Job drawing, mm, ordinate dimensions from the low corner. One solid piece. A direction names the side the tool comes from. Round coordinates to 2 decimals unless told otherwise and drop trailing zeros. Write each loop counter-clockwise with the first axis right and the second up, starting at its lowest first coordinate (ties: lowest second). Pieces come first, ordered by that corner, then holes.
1) Which spindle directions (+Z, -Z, +X, -X, +Y, -Y) get a long thin tool onto all of the face, cutting with end or side? Do the marked faces 1 and 2. Say none if no direction does.
2) Saw through at A-A on z = 20.2. Write the cut outline in (x, y), and give its area (3 significant figures).
3) Saw through at D-D on x = 1.75. Write the cut outline in (y, z), and give its area (3 significant figures).
4) Saw through at B-B on x = 10.75. Write the cut outline in (y, z), and give its area (3 significant figures).
5) Saw through at C-C on z = 9.25. Write the cut outline in (x, y), and give its area (3 significant figures).
6) Drill centre lines: L1, parallel to Z at x = 11, y = 0.9; L2, parallel to X at y = 0.2, z = 5.2; L3, parallel to Y at x = 13.5, z = 4.75. Where is each one in solid material? Low to high.
7) Flat gauge pins, fed straight in: pin 1 (1.1 mm diameter, centred on x = 4, z = 10, fed in from -Y); pin 2 (2 mm diameter, centred on y = 0.5, z = 21, fed in from -X); pin 3 (1.4 mm diameter, centred on x = 2, y = 3, fed in from +Z). Where does each tip first touch, or does it go through?
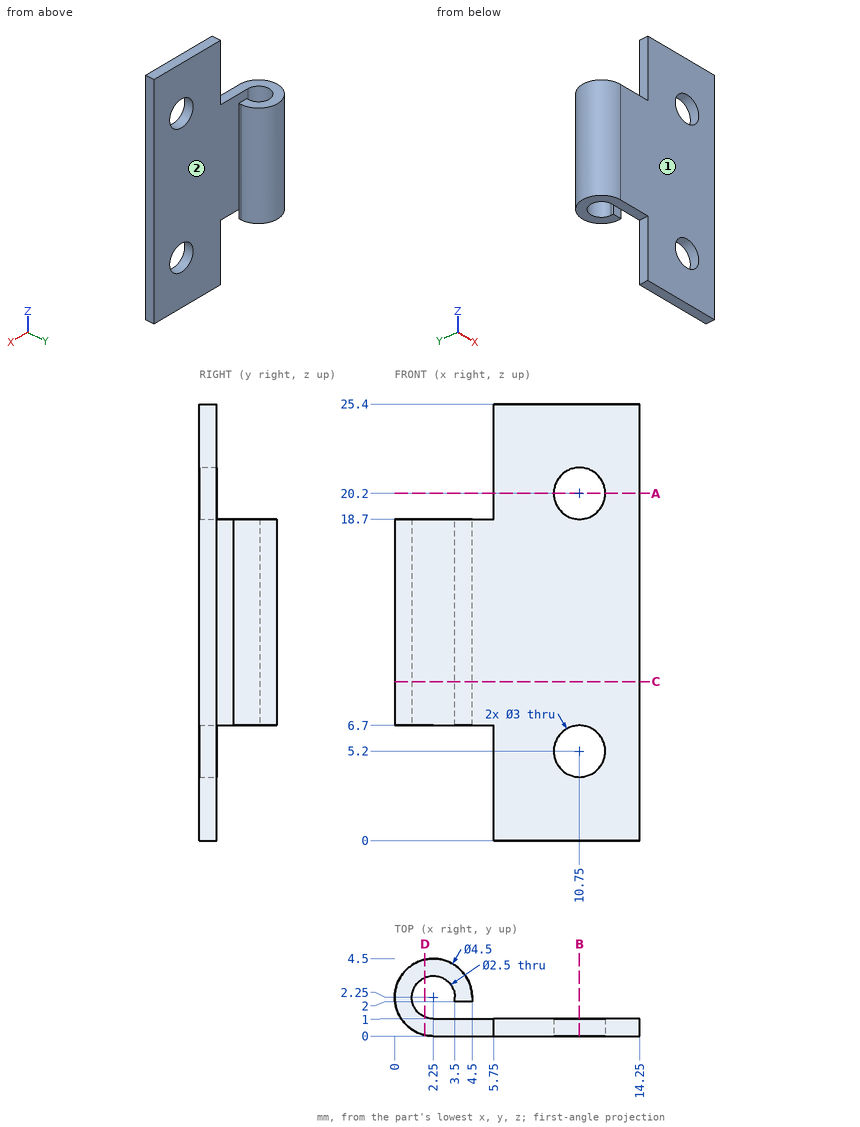
Completed:
1. face 1: +Z, -Z, +X, -X, -Y
1. face 2: +Z, -Z, +X
2. outline: (5.75, 0) - (9.25, 0) - (9.25, 1) - (5.75, 1) - close; (12.25, 0) - (14.25, 0) - (14.25, 1) - (12.25, 1) - close
2. area: 5.50 mm2
3. outline: (0.06, 6.7) - (1.1, 6.7) - (1.1, 18.7) - (0.06, 18.7) - close; (3.4, 6.7) - (4.44, 6.7) - (4.44, 18.7) - (3.4, 18.7) - close
3. area: 25.2 mm2
4. outline: (0, 0) - (1, 0) - (1, 3.7) - (0, 3.7) - close; (0, 6.7) - (1, 6.7) - (1, 18.7) - (0, 18.7) - close; (0, 21.7) - (1, 21.7) - (1, 25.4) - (0, 25.4) - close
4. area: 19.4 mm2
5. outline: (2.25, 0) - (14.25, 0) - (14.25, 1) - (2.25, 1) arc R1.25 cw (long way) to (3.5, 2.25) - (3.5, 2) - (4.5, 2) - (4.5, 2.25) arc R2.25 ccw (long way) to start
5. area: 20.5 mm2
6. L1: z = 0 to 3.72, 6.68 to 18.72, 21.68 to 25.4
6. L2: x = 5.75 to 9.25, 12.25 to 14.25
6. L3: y = 0 to 1
7. pin 1: stops at y = 0
7. pin 2: stops at x = 5.75
7. pin 3: stops at z = 18.7
